from build123d import *

# Parameters (mm, degrees)
SKETCH1_W           = 19
SKETCH1_H           = 39
SKETCH1_R           = 2.575
BOSS_EXTRUDE1_DEPTH = 3.8
SKETCH2_W           = 19
SKETCH2_H           = 9.5
SKETCH2_R           = 2.575
BOSS_EXTRUDE2_DEPTH = 9
SKETCH3_W           = 19
SKETCH3_H           = 39
SKETCH3_R           = 2.575
BOSS_EXTRUDE3_DEPTH = 4
FILLET1_R           = 8
FILLET2_R           = 3


with BuildPart() as part:
    # Sketch1 → Boss-Extrude1 (new body)
    with BuildSketch(Plane(origin=(0, 0, 0), x_dir=(-1, 0, 0), z_dir=(0, 1, 0))):
        Rectangle(SKETCH1_W, SKETCH1_H)
        with Locations(Location((0, 0, 0), (0, 0, 270))):
            Circle(SKETCH1_R, mode=Mode.SUBTRACT)
        with Locations(Location((0, 14.25, 0), (0, 0, 270))):
            Circle(SKETCH1_R, mode=Mode.SUBTRACT)
        with Locations(Location((0, -14.25, 0), (0, 0, 270))):
            Circle(SKETCH1_R, mode=Mode.SUBTRACT)
    extrude(amount=BOSS_EXTRUDE1_DEPTH)

    # Sketch2 → Boss-Extrude2 (add)
    # profile 1 of 2: a face of its own
    with BuildSketch(Plane(origin=(0, 3.8, 0), x_dir=(-1, 0, 0), z_dir=(0, 1, 0))):
        with Locations((0, 14.75)):
            Rectangle(SKETCH2_W, SKETCH2_H)
        with Locations(Location((0, 14.25, 0), (0, 0, 270))):
            Circle(SKETCH2_R, mode=Mode.SUBTRACT)
    # profile 2 of 2: a face of its own
    with BuildSketch(Plane(origin=(0, 3.8, 0), x_dir=(-1, 0, 0), z_dir=(0, 1, 0))):
        with Locations((0, -14.75)):
            Rectangle(SKETCH2_W, SKETCH2_H)
        with Locations(Location((0, -14.25, 0), (0, 0, 270))):
            Circle(SKETCH2_R, mode=Mode.SUBTRACT)
    extrude(amount=BOSS_EXTRUDE2_DEPTH)

    # Sketch3 → Boss-Extrude3 (add)
    with BuildSketch(Plane(origin=(0, 12.8, 0), x_dir=(-1, 0, 0), z_dir=(0, 1, 0))):
        Rectangle(SKETCH3_W, SKETCH3_H)
        with Locations(Location((0, 14.25, 0), (0, 0, 270))):
            Circle(SKETCH3_R, mode=Mode.SUBTRACT)
        with Locations(Location((0, 0, 0), (0, 0, 270))):
            Circle(SKETCH3_R, mode=Mode.SUBTRACT)
        with Locations(Location((0, -14.25, 0), (0, 0, 270))):
            Circle(SKETCH3_R, mode=Mode.SUBTRACT)
    extrude(amount=BOSS_EXTRUDE3_DEPTH)

    # Fillet1
    fillet1_edges = [part.edges().sort_by_distance(p)[0] for p in [
        (-9.5, 8.4, -19.5),
        (9.5, 8.4, -19.5),
        (9.5, 8.4, 19.5),
        (-9.5, 8.4, 19.5),
    ]]
    fillet(fillet1_edges, radius=FILLET1_R)

    # Fillet2
    # the kernel refuses this fillet: 3 mm, written as the material it takes off along each edge
    with BuildSketch(Plane(origin=(9.5, 3.8, 10), x_dir=(-0.09406475637410622, 0, 0.9955660809852251), z_dir=(0, 1, 0)), Plane(origin=(-9.5, 3.8, -10), x_dir=(0.09406475637410011, 0, -0.9955660809852258), z_dir=(0, 1, 0))) as fillet2_piece_1:
        with BuildLine():
            CenterArc((3.290556001, -2.933786817), FILLET2_R, 77.939890127, 107.457603124)
            Line((0.303857758, -3.215981087), (0.005187934, -3.244200514))
            Line((0.005187934, -3.244200514), (-0.298669824, -0.028219427))
            Line((-0.298669824, -0.028219427), (-0.028219427, 0.298669824))
            ThreePointArc((-0.028219427, 0.298669824), (1.465129695, 0.439766959), (3.980050628, 0.293378682))
            Line((3.980050628, 0.293378682), (3.917369298, 0))
        make_face()
    extrude(amount=9, mode=Mode.SUBTRACT)
    with BuildSketch(Plane(origin=(-9.5, 3.8, 10), x_dir=(0.09406475637410577, 0, 0.9955660809852253), z_dir=(0, 1, 0)), Plane(origin=(9.5, 3.8, -10), x_dir=(-0.09406475637410053, 0, -0.9955660809852258), z_dir=(0, 1, 0))) as fillet2_piece_2:
        with BuildLine():
            CenterArc((3.290556001, 2.933786817), FILLET2_R, 174.602506749, 107.457603124)
            Line((0.303857758, 3.215981087), (0.005187934, 3.244200514))
            Line((0.005187934, 3.244200514), (-0.298669824, 0.028219427))
            Line((-0.298669824, 0.028219427), (-0.028219427, -0.298669824))
            ThreePointArc((-0.028219427, -0.298669824), (1.465129695, -0.439766959), (3.980050628, -0.293378682))
            Line((3.980050628, -0.293378682), (3.917369298, 0))
        make_face()
    extrude(amount=9, mode=Mode.SUBTRACT)


solid = part.part
For this review, take the finished solid that the model builds, in its own axes (mm). A direction names the side the tool comes from. Give positions to 0.01 mm unless a question says otherwise; leave off trailing zeros. Loops run counter-clockwise (first coordinate to the right, second up) from the corner with the lowest first, then second, coordinate; pieces in that order, holes last. Notation, with made-up numbers: (64, 12.5) -> (111, 12.5) arc R11 cw to (111, 33.5) -> close; hole circle Ø5 at (28.25, -23). An arc over 180 degrees is marked (long way). One line per question, with ' | ' between items.
1) We need section C-C (x = 0). Write out the cut boundary in (y, z) (3 decimals).
Resolved:
outline: (0, -19.5) -> (16.8, -19.5) -> (16.8, -16.825) -> (0, -16.825) -> close; (0, -11.675) -> (16.8, -11.675) -> (16.8, -2.575) -> (12.8, -2.575) -> (12.8, -10) -> (3.8, -10) -> (3.8, -2.575) -> (0, -2.575) -> close; (0, 2.575) -> (3.8, 2.575) -> (3.8, 10) -> (12.8, 10) -> (12.8, 2.575) -> (16.8, 2.575) -> (16.8, 11.675) -> (0, 11.675) -> close; (0, 16.825) -> (16.8, 16.825) -> (16.8, 19.5) -> (0, 19.5) -> close
2) For faces 4 (the cylindrical face through (8.711, 8.237, 11.257)), 5 (the cylindrical face through (-8.711, 8.237, -11.257)), 6 (the flat face through (0, 8, 10)), list the 3-axis set-ups (+Z, -Z, +X, -X, +Y, -Y) from which the entire face can be reached by the end or side of a thin tool; tool diameter is ignored.
Resolved:
face 4: +X | face 5: -X | face 6: +X, -X
3) We need section B-B (y = 3.25). Write out the cut boundary in (x, z) (3 decimals).
Resolved:
outline: (-9.5, -11.5) arc R8 ccw to (-1.5, -19.5) -> (1.5, -19.5) arc R8 ccw to (9.5, -11.5) -> (9.5, 11.5) arc R8 ccw to (1.5, 19.5) -> (-1.5, 19.5) arc R8 ccw to (-9.5, 11.5) -> close; hole circle Ø5.15 at (0, -14.25); hole circle Ø5.15 at (0, 0); hole circle Ø5.15 at (0, 14.25)
4) We need section D-D (y = 5.25). Write out the cut boundary in (x, z) (3 decimals).
Resolved:
outline: (-9.132, -13.9) arc R8 ccw to (-1.5, -19.5) -> (1.5, -19.5) arc R8 ccw to (9.132, -13.9) arc R3 ccw to (6.27, -10) -> (-6.27, -10) arc R3 ccw to start; (-9.132, 13.9) arc R3 ccw to (-6.27, 10) -> (6.27, 10) arc R3 ccw to (9.132, 13.9) arc R8 ccw to (1.5, 19.5) -> (-1.5, 19.5) arc R8 ccw to start; hole circle Ø5.15 at (0, -14.25); hole circle Ø5.15 at (0, 14.25)
5) The part is to be moulded in two halves that separate along Y. For faces 1 (the flat face through (0, 0, -4)), 2 (the cylindrical face through (8.66, 8.24, -11.19)), 3 (the flat face through (-9.5, 15, 0)), say which applies: +Y half, -Y half, draft (parallel to the pull), parting line (faces both ways), or undercut.
Resolved:
face 1: -Y half | face 2: undercut | face 3: draft
6) Insertion check: pin 1 Ø1 at (y, z) = (2, 13.5) entering from -X. The pin has a flat end and moves straight along its axis. Give the tip position at first contact, or say it passes through.
Resolved:
pin 1: stops at x = -9.36
7) We need section A-A (z = 3). Write out the cut boundary in (x, y).
Resolved:
outline: (-9.5, 0) -> (9.5, 0) -> (9.5, 3.8) -> (-9.5, 3.8) -> close; (-9.5, 12.8) -> (9.5, 12.8) -> (9.5, 16.8) -> (-9.5, 16.8) -> close
8) To check wall thickness, follow probe 1 along X at (y, z) = (13.8, 0) (3 decimals); probe 2 along Y at (x, z) = (3, 4.5); probe 3 along Z at (x, y) = (-2.25, 1.25). State the ranges of each line that lie inside material, in increasing order.
Resolved:
probe 1: x = -9.5 to -2.575, 2.575 to 9.5 | probe 2: y = 0 to 3.8, 12.8 to 16.8 | probe 3: z = -19.46 to -15.5, -13 to -1.25, 1.25 to 13, 15.5 to 19.46
